Check sheet for the modelled part. Datum: model origin and axes. Units: mm. A direction names the side the tool comes from. Round coordinates to 2 decimals unless told otherwise and drop trailing zeros. Order: outer loops, then holes, each group sorted by start corner. A loop starts at its lowest first (then second) coordinate and runs counter-clockwise, first axis right, second up. Notation, with made-up numbers: (56, 74) -> (68, 74) arc R20 ccw to (68, 78) -> close; hole circle Ø4 at (-5, -0.5). An arc over 180 degrees is marked (long way). Answer in a Markdown table with one row per item. Add a question column.
1. Sectioned sample at A-A, the plane x = -353.5. Record the boundary of the cut face in (y, z).
2. Access from +Z, -Z, +X, -X, +Y, -Y to the whole of each face (thin tool, end or side, straight path). Record for faces 4 (the flat face through (13, -25, 0)), 5 (the flat face through (-537, -25, 0)), 6 (the flat face through (-518, -30, 0)), 7 (the flat face through (7, -22, 0)), 8 (the flat face through (507, -2, 0)).
3. Depth check by flat-ended pin: P1, Ø9.5, axis at x = 462, z = 10, coming from the -Y side; P2, Ø16, axis at x = -522, z = 10, coming from the +Y side; P3, Ø10, axis at x = 292.5, z = -6.5, coming from the -Y side. Enter the tip coordinate at first touch or a pass-through.
4. Draft check along Y on faces 1 (the flat face through (7, -13, -22)), 2 (the flat face through (-7, 0, 0)), 3 (the flat face through (-38, -15, 25)). Enter one of: +Y half, -Y half, draft (parallel to the pull), parting line (faces both ways), or undercut.
5. Material ranges on L1, parallel to Z at x = 462, y = -24.2; L2, parallel to Y at x = 58.5, z = -10; L3, parallel to X at y = -24.25, z = 8, recorded low to high. Write a range as from..to.
6. Sectioned sample at B-B, the plane y = -15.25. Record the boundary of the cut face in (x, z), then the cut area to 3 significant figures.
```python
from build123d import *

# Parameters (mm, degrees)
F0_W     = 1014
F0_H     = 50
F1_DEPTH = 25
F2_R     = 8
F3_DEPTH = 25
F4_W     = 19
F4_H     = 44
F5_DEPTH = 1014
F6_W     = 100
F6_H     = 50
F6_R     = 5
F7_DEPTH = 5


with BuildPart() as f1:
    # F0 (on Front) → F1 (new body)
    with BuildSketch(Plane.XZ):
        Rectangle(F0_W, F0_H)
    extrude(amount=F1_DEPTH)

    # F2 (on face) → F3 (cut)
    with BuildSketch(Plane.XZ.offset(25)):
        with Locations((462, 10)):
            Circle(F2_R)
        with Locations((462, -10)):
            Circle(F2_R)
        with Locations((492, 10)):
            Circle(F2_R)
        with Locations((492, -10)):
            Circle(F2_R)
    extrude(amount=-F3_DEPTH, mode=Mode.SUBTRACT)

    # F4 (on face) → F5 (cut)
    with BuildSketch(Plane.YZ.offset(507)):
        with Locations((-12.5, 0)):
            Rectangle(F4_W, F4_H)
    extrude(amount=-F5_DEPTH, mode=Mode.SUBTRACT)

    # F6 (on face) → F7 (join)
    with BuildSketch(Plane.XZ.offset(25)):
        with Locations((-517, 0)):
            Rectangle(F6_W, F6_H)
        with Locations((-552, -10)):
            Circle(F6_R, mode=Mode.SUBTRACT)
        with Locations((-522, -10)):
            Circle(F6_R, mode=Mode.SUBTRACT)
        with Locations((-552, 10)):
            Circle(F6_R, mode=Mode.SUBTRACT)
        with Locations((-522, 10)):
            Circle(F6_R, mode=Mode.SUBTRACT)
    extrude(amount=F7_DEPTH)


solid = f1.part
```
Answer key:
| question | item | result |
|---|---|---|
| 1 | outline | (-25, -25) -> (0, -25) -> (0, 25) -> (-25, 25) -> close; hole (-22, -22) -> (-3, -22) -> (-3, 22) -> (-22, 22) -> close |
| 2 | face 4 | +Z, -Z, +X, -Y |
| 2 | face 5 | +Z, -Z, -X, +Y |
| 2 | face 6 | +Z, -Z, +X, -X, -Y |
| 2 | face 7 | +X, -X |
| 2 | face 8 | +Z, -Z, +X, +Y, -Y |
| 3 | P1 | passes through |
| 3 | P2 | stops at y = -25 |
| 3 | P3 | stops at y = -25 |
| 4 | face 1 | undercut |
| 4 | face 2 | +Y half |
| 4 | face 3 | draft |
| 5 | L1 | z = -25..-18, -2..2, 18..25 |
| 5 | L2 | y = -25..-22, -3..0 |
| 5 | L3 | x = -507..454.25, 469.75..484.25, 499.75..507 |
| 6 | outline | (-507, -25) -> (507, -25) -> (507, -22) -> (-507, -22) -> close; (-507, 22) -> (507, 22) -> (507, 25) -> (-507, 25) -> close |
| 6 | area | 6,080 mm² |
